Build history of the part. All positions in model axes, mm. Face numbers are marked on the shaded views. A direction names the side the tool comes from. Give positions to 0.01 mm unless a question says otherwise; leave off trailing zeros. Order: outer loops, then holes, each group sorted by start corner. A loop starts at its lowest first (then second) coordinate and runs counter-clockwise, first axis right, second up. Notation, with made-up numbers: (-15.75, 63) - (34.25, 63) arc R24 ccw to (34.25, 89) - close; hole circle Ø11 at (-21, 51). An arc over 180 degrees is marked (long way). Use a Markdown table: item, result.
from build123d import *

# Parameters (mm, degrees)
SKETCH1_W           = 100
SKETCH1_H           = 40
BOSS_EXTRUDE1_DEPTH = 175
SKETCH2_W           = 90
SKETCH2_H           = 165
CUT_EXTRUDE1_DEPTH  = 30
SKETCH18_R          = 7
SKETCH18_R_2        = 9
CUT_EXTRUDE9_DEPTH  = 10
BOSS_EXTRUDE3_DEPTH = 6
SKETCH27_W          = 2
SKETCH27_H          = 3
CUT_EXTRUDE13_DEPTH = 92
SKETCH28_W          = 2
SKETCH28_H          = 3
CUT_EXTRUDE14_DEPTH = 92
SKETCH29_W          = 165
SKETCH29_H          = 3
CUT_EXTRUDE15_DEPTH = 2


with BuildPart() as part:
    # Sketch1 → Boss-Extrude1 (new body)
    with BuildSketch(Plane.XY):
        with Locations((6.252485089, -6.669980119)):
            Rectangle(SKETCH1_W, SKETCH1_H)
    extrude(amount=BOSS_EXTRUDE1_DEPTH)

    # Sketch2 → Cut-Extrude1 (cut)
    with BuildSketch(Plane(origin=(0, 13.330019881, 0), x_dir=(1, 0, 0), z_dir=(0, 1, 0))):
        with Locations((6.252485089, -87.5)):
            Rectangle(SKETCH2_W, SKETCH2_H)
    extrude(amount=-CUT_EXTRUDE1_DEPTH, mode=Mode.SUBTRACT)

    # Sketch18 → Cut-Extrude9 (cut)
    with BuildSketch(Plane.XY):
        with Locations((6.252485089, -1.669980119)):
            Circle(SKETCH18_R)
        with Locations((36.752485089, -1.669980119)):
            Circle(SKETCH18_R_2)
        with Locations((-24.247514911, -1.669980119)):
            Circle(SKETCH18_R_2)
    extrude(amount=CUT_EXTRUDE9_DEPTH, mode=Mode.SUBTRACT)

    # Sketch26 → Boss-Extrude3 (add)
    with BuildSketch(Plane(origin=(0, 13.330019881, 0), x_dir=(1, 0, 0), z_dir=(0, 1, 0))):
        Polygon((51.252485089, -5), (-38.747514911, -5), (-38.747514911, -170), (51.252485089, -170), (51.252485089, -175), (-43.747514911, -175), (-43.747514911, 0), (51.252485089, 0), align=None)
    extrude(amount=BOSS_EXTRUDE3_DEPTH)

    # Sketch27 → Cut-Extrude13 (cut)
    with BuildSketch(Plane(origin=(51.252485089, 0, 0), x_dir=(0, 0, -1), z_dir=(1, 0, 0))):
        with Locations((-171, 14.830019881)):
            Rectangle(SKETCH27_W, SKETCH27_H)
    extrude(amount=-CUT_EXTRUDE13_DEPTH, mode=Mode.SUBTRACT)

    # Sketch28 → Cut-Extrude14 (cut)
    with BuildSketch(Plane(origin=(51.252485089, 0, 0), x_dir=(0, 0, -1), z_dir=(1, 0, 0))):
        with Locations((-4, 14.830019881)):
            Rectangle(SKETCH28_W, SKETCH28_H)
    extrude(amount=-CUT_EXTRUDE14_DEPTH, mode=Mode.SUBTRACT)

    # Sketch29 → Cut-Extrude15 (cut)
    with BuildSketch(Plane(origin=(-38.747514911, 0, 0), x_dir=(0, 0, -1), z_dir=(1, 0, 0))):
        with Locations((-87.5, 14.830019881)):
            Rectangle(SKETCH29_W, SKETCH29_H)
    extrude(amount=-CUT_EXTRUDE15_DEPTH, mode=Mode.SUBTRACT)


solid = part.part
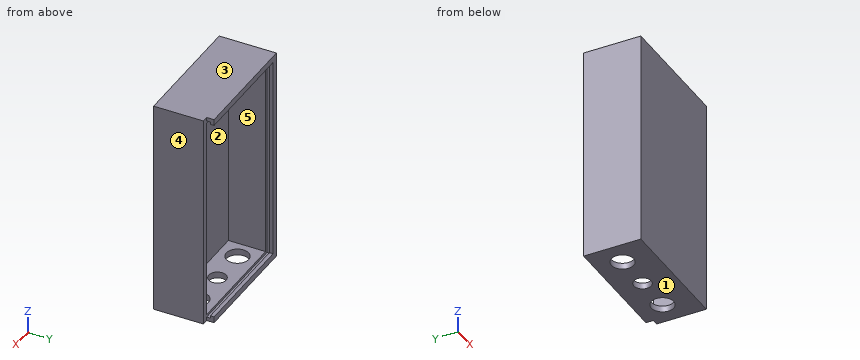
1) Slice it at D-D (x = -20). Write the cut outline in (y, z).
Computed:
| item | result |
|---|---|
| outline | (-26.67, 0) - (-9.6, 0) - (-9.6, 5) - (-16.67, 5) - (-16.67, 170) - (13.33, 170) - (13.33, 172) - (16.33, 172) - (16.33, 170) - (19.33, 170) - (19.33, 175) - (-26.67, 175) - close; (6.26, 0) - (19.33, 0) - (19.33, 5) - (16.33, 5) - (16.33, 3) - (13.33, 3) - (13.33, 5) - (6.26, 5) - close |
2) Wall check: line 1 (Z direction, x = 20.5, y = -13); line 2 (X direction, y = 12.5, z = 28); line 3 (Y direction, x = -24.5, z = 76.5). Give the ranges that are in metal, low to high. Write a range as from..to.
Computed:
| item | result |
|---|---|
| line 1 | z = 0..5, 170..175 |
| line 2 | x = -43.75..-38.75, 51.25..56.25 |
| line 3 | y = -26.67..-16.67 |
3) Tool access for the marked faces 1 and 2: list every direction of +Z, -Z, +X, -X, +Y, -Y with a clear straight run to the whole face (end or side of a thin tool).
Computed:
| item | result |
|---|---|
| face 1 | -Z, +X, -X, +Y, -Y |
| face 2 | +Y |
4) Two-plate mould, pull along Z, no slides. Class the marked faces 3, 4 and 5: +Z half, -Z half, draft (parallel to the pull), parting line (faces both ways), or undercut.
Computed:
| item | result |
|---|---|
| face 3 | +Z half |
| face 4 | draft |
| face 5 | undercut |
5) Slice it at A-A (y = 9). Write the cut outline in (x, z), and give its area (3 significant figures).
Computed:
| item | result |
|---|---|
| outline | (-43.75, 0) - (56.25, 0) - (56.25, 175) - (-43.75, 175) - close; hole (-38.75, 5) - (51.25, 5) - (51.25, 170) - (-38.75, 170) - close |
| area | 2,650 mm² |
6) Slice it at B-B (y = -5). Write the cut outline in (x, z), and give its area (3 significant figures).
Computed:
| item | result |
|---|---|
| outline | (-43.75, 0) - (-32.61, 0) - (-32.61, 5) - (-38.75, 5) - (-38.75, 170) - (51.25, 170) - (51.25, 5) - (45.11, 5) - (45.11, 0) - (56.25, 0) - (56.25, 175) - (-43.75, 175) - close; (-15.89, 0) - (0.1, 0) - (0.1, 5) - (-15.89, 5) - close; (12.41, 0) - (28.39, 0) - (28.39, 5) - (12.41, 5) - close |
| area | 2,420 mm² |
7) Pin check, flat tips, straight feed: P1, Ø1.5, axis at y = 16, z = 173.5, coming from the +X side; P2, Ø6, axis at x = -2, z = 132, coming from the +Y side; P3, Ø1.5, axis at y = 18.5, z = 94.5, coming from the +X side. Stop position of each tip, or through.
Computed:
| item | result |
|---|---|
| P1 | stops at x = 51.25 |
| P2 | stops at y = -16.67 |
| P3 | stops at x = -38.75 |
8) Slice it at C-C (z = 125). Write the cut outline in (x, y).
Computed:
| item | result |
|---|---|
| outline | (-43.75, -26.67) - (56.25, -26.67) - (56.25, 13.33) - (51.25, 13.33) - (51.25, -16.67) - (-38.75, -16.67) - (-38.75, 13.33) - (-40.75, 13.33) - (-40.75, 16.33) - (-38.75, 16.33) - (-38.75, 19.33) - (-43.75, 19.33) - close |
